Design review of the part built by this model. Coordinates are the model's own, in mm. A direction names the side the tool comes from. Give positions to 0.01 mm unless a question says otherwise; leave off trailing zeros. Write each loop counter-clockwise with the first axis right and the second up, starting at its lowest first coordinate (ties: lowest second). Pieces come first, ordered by that corner, then holes. Notation, with made-up numbers: M -6,-5.5 L 0,-5.5 A24 ccw 0,20.5 Z; hole C 77,19.25 d9. An arc over 180 degrees is marked long. Answer in a Markdown table with one row per item.
```python
from build123d import *

# Parameters (mm, degrees)
F0_W           = 21
F0_H           = 5
F0_H_2         = 16.25
F1_DEPTH       = 13
F2_D           = 12.25
F2_CBORE_D     = 16.25
F2_CBORE_DEPTH = 3.1
F4_D           = 16.25
F4_DEPTH       = 4
F4_TIP         = 4.8819925296
F5_D           = 18.1


with BuildPart() as f1:
    # F0 (on Top) → F1 (new body)
    with BuildSketch(Plane.XY):
        with Locations((-10.5, -2.5)):
            Rectangle(F0_W, F0_H)
        with Locations((10.5, -2.5)):
            Rectangle(F0_W, F0_H)
        Polygon((-21, -5), (-21, 0), (-26, 0), (-42, 0), (-42, -5), align=None)
        Polygon((26, 0), (21, 0), (21, -5), (42, -5), (42, 0), align=None)
        with Locations((-31.5, -13.125)):
            Rectangle(F0_W, F0_H_2)
        with Locations((31.5, -13.125)):
            Rectangle(F0_W, F0_H_2)
        Polygon((0, -28.25), (0, -21.25), (-21, -21.25), (-21, -28.25), (-6, -28.25), align=None)
        Polygon((21, -21.25), (0, -21.25), (0, -28.25), (6, -28.25), (21, -28.25), align=None)
        Polygon((-21, -28.25), (-21, -21.25), (-42, -21.25), (-42, -28.25), (-36, -28.25), align=None)
        Polygon((42, -21.25), (21, -21.25), (21, -28.25), (36, -28.25), (42, -28.25), align=None)
        with BuildLine():
            Line((-6, -28.25), (-21, -28.25))
            Line((-21, -28.25), (-36, -28.25))
            Line((-36, -28.25), (-36, -36.6772486205))
            ThreePointArc((-36, -36.6772486205), (-21, -43.4484920652), (-6, -36.6772486205))
            Line((-6, -36.6772486205), (-6, -28.25))
        make_face()
        with BuildLine():
            Line((36, -28.25), (21, -28.25))
            Line((21, -28.25), (6, -28.25))
            Line((6, -28.25), (6, -36.6772486205))
            ThreePointArc((6, -36.6772486205), (21, -43.4484920652), (36, -36.6772486205))
            Line((36, -36.6772486205), (36, -28.25))
        make_face()
        with Locations((10.5, -13.125)):
            Rectangle(F0_W, F0_H_2)
        with Locations((-10.5, -13.125)):
            Rectangle(F0_W, F0_H_2)
    extrude(amount=F1_DEPTH)

    # F2 (through all)
    with Locations(Plane(origin=(0, 0, 0), x_dir=(1, 0, 0), z_dir=(0, 0, -1))):
        with Locations((21, 21.25), (-21, 21.25)):
            CounterBoreHole(F2_D / 2, F2_CBORE_D / 2, F2_CBORE_DEPTH)

    # F4
    with Locations(Plane.XY.offset(13)):
        with Locations((-21, -21.25), (21, -21.25)):
            Hole(F4_D / 2, depth=F4_DEPTH)
            with Locations((0, 0, -(F4_DEPTH + F4_TIP / 2))):  # 118° drill point
                Cone(0, F4_D / 2, F4_TIP, mode=Mode.SUBTRACT)

    # F5 (through all)
    with Locations(Plane(origin=(0, 0, 0), x_dir=(1, 0, 0), z_dir=(0, 0, -1))):
        with Locations((0, 13.125)):
            Hole(F5_D / 2)


solid = f1.part
```
1) The part is to be moulded in two halves that separate along X. For faces 1 (the face through (36, -33, 6)), 2 (the face through (2, -4.3, 6.6)), 3 (the face through (-36, -32, 6)), 4 (the face through (1, 0, 6)), say which applies: released by +X, released by -X, zero draft, split by the parting line, or undercut.
Geometry says:
| item | result |
|---|---|
| face 1 | released by +X |
| face 2 | undercut |
| face 3 | released by -X |
| face 4 | zero draft |
2) Add section B-B (z = 10.5). Count the separate pieces of the cut face and the enclosed holes in it, and give its area (3 significant figures).
Geometry says:
| item | result |
|---|---|
| separate pieces | 1 |
| enclosed holes | 3 |
| area | 2,490 mm^2 |
3) Add section A-A (x = 0). Write out the cut boundary in (y, z) (3 decimals).
Geometry says:
| item | result |
|---|---|
| outline | M -28.25,0 L -22.175,0 L -22.175,13 L -28.25,13 Z; M -4.075,0 L 0,0 L 0,13 L -4.075,13 Z |
4) For faces 5 (the face through (-15.01, -15.76, 10.97)), 6 (the face through (39, -28.25, 6)), 7 (the face through (6, -32, 6)), list the 3-axis set-ups (+Z, -Z, +X, -X, +Y, -Y) from which the entire face can be reached by the end or side of a thin tool; tool diameter is ignored.
Geometry says:
| item | result |
|---|---|
| face 5 | +Z |
| face 6 | +Z, -Z, +X, -Y |
| face 7 | +Z, -Z, -Y |
5) Add section C-C (y = -11). Write out the cut boundary in (x, z), and give its area (3 significant figures).
Geometry says:
| item | result |
|---|---|
| outline | M -42,0 L -8.8,0 L -8.8,13 L -42,13 Z; M 8.8,0 L 42,0 L 42,13 L 8.8,13 Z |
| area | 863 mm^2 |
6) Insertion check: P1, Ø4, axis at y = -33.5, z = 4.5, coming from the +X side; P2, Ø4, axis at y = -32, z = 7.5, coming from the -X side; P3, Ø6, axis at x = -1.5, z = 5, coming from the -Y side. Each pin has a flat end and moves straight along its axis. Give the tip position at first contact, or say it passes through.
Geometry says:
| item | result |
|---|---|
| P1 | x = 36 |
| P2 | x = -36 |
| P3 | y = -28.25 |
7) Add section D-D (x = -21). Write out the cut boundary in (y, z) (1 decimal).
Geometry says:
| item | result |
|---|---|
| outline | M -43.4,0 L -29.4,0 L -29.4,3.1 L -27.4,3.1 L -27.4,7.8 L -29.4,9 L -29.4,13 L -43.4,13 Z; M -15.1,3.1 L -13.1,3.1 L -13.1,0 L 0,0 L 0,13 L -13.1,13 L -13.1,9 L -15.1,7.8 Z |
8) To check wall thickness, follow probe 1 along X at (y, z) = (-21.25, 6.4) (3 decimals); probe 2 along Y at (x, z) = (-21, 5.5) (1 decimal); probe 3 along X at (y, z) = (-21.25, 11.95) (3 decimals). State the ranges of each line that lie inside material, in increasing order. Write a range as [from, to].
Geometry says:
| item | result |
|---|---|
| probe 1 | [-42, -27.125], [-14.875, -3.986], [3.986, 14.875], [27.125, 42] |
| probe 2 | [-43.4, -27.4], [-15.1, 0] |
| probe 3 | [-42, -29.125], [-12.875, -3.986], [3.986, 12.875], [29.125, 42] |
